CAD build for the part. Positions are in the model's coordinates, mm. Face numbers are marked on the shaded views. Round coordinates to 2 decimals unless told otherwise and drop trailing zeros.
from build123d import *

# Parameters (mm, degrees)
BOSS_EXTRUDE1_OUTLINE_R   = 62
BOSS_EXTRUDE1_OUTLINE_R_2 = 1.575
BOSS_EXTRUDE1_OUTLINE_R_3 = 56.5
BOSS_EXTRUDE1_DEPTH       = 33
BOSS_EXTRUDE2_START       = -5
SKETCH2_R                 = 56.5
SKETCH2_R_2               = 15
BOSS_EXTRUDE2_DEPTH       = 5
SKETCH3_R                 = 16.025
CUT_EXTRUDE1_DEPTH        = 4
SKETCH4_W                 = 8
SKETCH4_H                 = 10
CUT_EXTRUDE2_DEPTH        = 190.339520636
FILLET1_R                 = 1
SKETCH5_R                 = 2.1
CUT_EXTRUDE3_DEPTH        = 5
SKETCH6_W                 = 30
SKETCH6_H                 = 10
CUT_EXTRUDE4_DEPTH        = 4
FILLET2_R                 = 1
SKETCH7_R                 = 2.1
CUT_EXTRUDE5_DEPTH        = 10


# Read off the part's stored shape, not the designer's step: Boss-Extrude1
with BuildPart() as part:
    # Boss-Extrude1 outline → Boss-Extrude1 (new body)
    with BuildSketch(Plane(origin=(0, 0, -63.995840519), x_dir=(-1, 0, 0), z_dir=(0, 0, -1))):
        with Locations((-89.072792821, 47.25870832)):
            Circle(BOSS_EXTRUDE1_OUTLINE_R)
        with Locations((-127.709576124, 2.669483434)):
            Circle(BOSS_EXTRUDE1_OUTLINE_R_2, mode=Mode.SUBTRACT)
        with Locations((-97.469368279, -11.14075675)):
            Circle(BOSS_EXTRUDE1_OUTLINE_R_2, mode=Mode.SUBTRACT)
        with Locations((-145.682878264, 30.636487467)):
            Circle(BOSS_EXTRUDE1_OUTLINE_R_2, mode=Mode.SUBTRACT)
        with Locations((-64.563307054, -6.409579405)):
            Circle(BOSS_EXTRUDE1_OUTLINE_R_2, mode=Mode.SUBTRACT)
        with Locations((-39.438834384, 15.360900091)):
            Circle(BOSS_EXTRUDE1_OUTLINE_R_2, mode=Mode.SUBTRACT)
        with Locations((-145.682878264, 63.880929174)):
            Circle(BOSS_EXTRUDE1_OUTLINE_R_2, mode=Mode.SUBTRACT)
        with Locations((-127.709576124, 91.847933207)):
            Circle(BOSS_EXTRUDE1_OUTLINE_R_2, mode=Mode.SUBTRACT)
        with Locations((-97.469368279, 105.658173391)):
            Circle(BOSS_EXTRUDE1_OUTLINE_R_2, mode=Mode.SUBTRACT)
        with Locations((-89.072792821, 47.25870832)):
            Circle(BOSS_EXTRUDE1_OUTLINE_R_3, mode=Mode.SUBTRACT)
        with Locations((-30.072792821, 47.25870832)):
            Circle(BOSS_EXTRUDE1_OUTLINE_R_2, mode=Mode.SUBTRACT)
        with Locations((-64.563307054, 100.926996046)):
            Circle(BOSS_EXTRUDE1_OUTLINE_R_2, mode=Mode.SUBTRACT)
        with Locations((-39.438834384, 79.15651655)):
            Circle(BOSS_EXTRUDE1_OUTLINE_R_2, mode=Mode.SUBTRACT)
    extrude(amount=BOSS_EXTRUDE1_DEPTH)

    # Sketch2 → Boss-Extrude2 (add)
    with BuildSketch(Plane(origin=(0, 0, -96.995840519), x_dir=(-1, 0, 0), z_dir=(0, 0, -1)).offset(BOSS_EXTRUDE2_START)):
        with Locations((-89.072792821, 47.25870832)):
            Circle(SKETCH2_R)
        with Locations((-89.072792821, 47.25870832)):
            Circle(SKETCH2_R_2, mode=Mode.SUBTRACT)
    extrude(amount=BOSS_EXTRUDE2_DEPTH)

    # Sketch3 → Cut-Extrude1 (cut)
    with BuildSketch(Plane.XY.offset(-91.995840519)):
        with Locations((89.072792821, 47.25870832)):
            Circle(SKETCH3_R)
    extrude(amount=-CUT_EXTRUDE1_DEPTH, mode=Mode.SUBTRACT)

    # Sketch4 → Cut-Extrude2 (cut, through all)
    with BuildSketch(Plane.XY.offset(-63.995840519)):
        with Locations((151.072792821, 47.25870832)):
            Rectangle(SKETCH4_W, SKETCH4_H)
    extrude(amount=-CUT_EXTRUDE2_DEPTH, mode=Mode.SUBTRACT)

    # Fillet1
    fillet1_edges = [part.edges().sort_by_distance(p)[0] for p in [
        (150.870851043, 42.25870832, -80.495840519),
        (150.870851043, 52.25870832, -80.495840519),
    ]]
    fillet(fillet1_edges, radius=FILLET1_R)

    # Sketch5 → Cut-Extrude3 (cut)
    with BuildSketch(Plane(origin=(0, 0, -96.995840519), x_dir=(-1, 0, 0), z_dir=(0, 0, -1))):
        with Locations((-117.357064069, 75.542979568)):
            Circle(SKETCH5_R)
        with Locations((-60.788521574, 75.542979568)):
            Circle(SKETCH5_R)
        with Locations((-60.788521574, 18.974437073)):
            Circle(SKETCH5_R)
        with Locations((-117.357064069, 18.974437073)):
            Circle(SKETCH5_R)
    extrude(amount=-CUT_EXTRUDE3_DEPTH, mode=Mode.SUBTRACT)

    # Sketch6 → Cut-Extrude4 (cut)
    with BuildSketch(Plane(origin=(0, 0, -96.995840519), x_dir=(-1, 0, 0), z_dir=(0, 0, -1))):
        with Locations((-132.072792821, 47.25870832)):
            Rectangle(SKETCH6_W, SKETCH6_H)
    extrude(amount=-CUT_EXTRUDE4_DEPTH, mode=Mode.SUBTRACT)

    # Fillet2
    fillet2_edges = [part.edges().sort_by_distance(p)[0] for p in [
        (147.072792821, 47.25870832, -92.995840519),
        (117.072792821, 47.25870832, -92.995840519),
        (117.072792821, 47.25870832, -96.995840519),
        (133.424893243, 42.25870832, -96.995840519),
        (86.019909262, -14.666083985, -96.995840519),
        (133.424893243, 52.25870832, -96.995840519),
        (150.518060684, 52.587277258, -96.995840519),
        (150.518060684, 41.930139383, -96.995840519),
    ]]
    fillet(fillet2_edges, radius=FILLET2_R)

    # Sketch7 → Cut-Extrude5 (cut)
    with BuildSketch(Plane.XY.offset(-63.995840519)):
        with Locations((30.072792821, 47.25870832)):
            Circle(SKETCH7_R)
        with Locations((39.438834384, 79.15651655)):
            Circle(SKETCH7_R)
        with Locations((64.563307054, 100.926996046)):
            Circle(SKETCH7_R)
        with Locations((97.469368279, 105.658173391)):
            Circle(SKETCH7_R)
        with Locations((127.709576124, 91.847933207)):
            Circle(SKETCH7_R)
        with Locations((145.682878264, 63.880929174)):
            Circle(SKETCH7_R)
        with Locations((145.682878264, 30.636487467)):
            Circle(SKETCH7_R)
        with Locations((127.709576124, 2.669483434)):
            Circle(SKETCH7_R)
        with Locations((97.469368279, -11.14075675)):
            Circle(SKETCH7_R)
        with Locations((64.563307054, -6.409579405)):
            Circle(SKETCH7_R)
        with Locations((39.438834384, 15.360900091)):
            Circle(SKETCH7_R)
    extrude(amount=-CUT_EXTRUDE5_DEPTH, mode=Mode.SUBTRACT)


solid = part.part
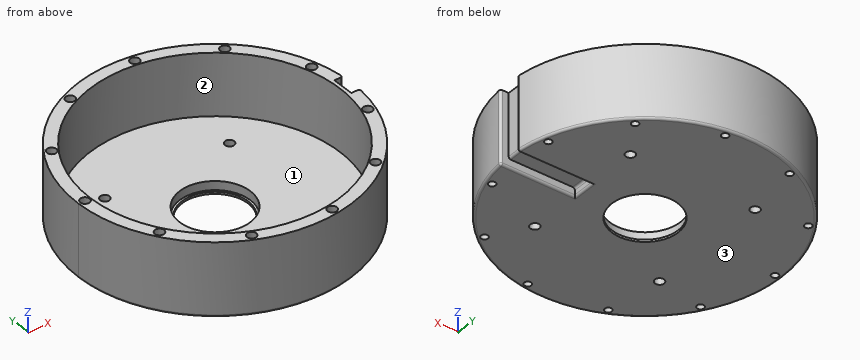
Item 1: Cut at A-A (z = -71.5). State how many separate pieces and enclosed holes the cut face has, plus the area to 3 significant figures.
Verdict:
separate pieces: 1
enclosed holes: 12
area: 1,860 mm2
Item 2: Wall check: L1, parallel to Z at x = 54, y = 68; L2, parallel to X at y = 14.5, z = -80; L3, parallel to X at y = 76, z = -95. Give the ranges that are in metal, low to high.
Verdict:
L1: z = -97 to -92
L2: x = 36.43 to 38.12, 40.76 to 43.04, 135.11 to 141.71
L3: x = 34.14 to 58.74, 62.84 to 115.31, 119.41 to 144.01
Item 3: Flat gauge pins, fed straight in: P1, Ø3.5, axis at x = 64.56, y = -6.41, coming from the -Z side; P2, Ø12, axis at y = 84.5, z = -68, coming from the +X side; P3, Ø10, axis at x = 79.5, z = -73, coming from the +Y side; P4, Ø3.5, axis at x = 39.44, y = 79.16, coming from the +Z side. Where does each tip first touch, or does it go through?
Verdict:
P1: stops at z = -97
P2: stops at x = 142.63
P3: stops at y = 109.09
P4: stops at z = -74
Item 4: Mould opens along Y. For the marked faces 1, 2 and 3 say: released by +Y, released by -Y, zero draft, split by the parting line, or undercut.
Verdict:
face 1: undercut
face 2: undercut
face 3: zero draft
